Design review of the part built by this model. Coordinates are the model's own, in mm. Face numbers are marked on the shaded views. A direction names the side the tool comes from. Give positions to 0.01 mm unless a question says otherwise; leave off trailing zeros. Write each loop counter-clockwise with the first axis right and the second up, starting at its lowest first coordinate (ties: lowest second). Pieces come first, ordered by that corner, then holes. Notation, with made-up numbers: (69, 37) -> (113, 37) arc R32 cw to (113, 75) -> close; hole circle Ø5 at (60.25, 86). An arc over 180 degrees is marked (long way). Use CSV: the item, a comma, the result in double quotes.
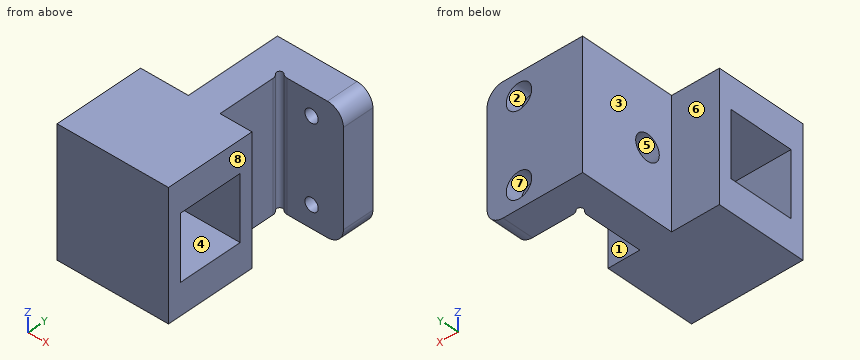
```python
from build123d import *

# Parameters (mm, degrees)
DODANIE_WYCI_GNI_CIE1_DEPTH = 40
SZKIC7_R                    = 4
WYTNIJ_WYCI_GNI_CIE2_DEPTH  = 5
SZKIC8_R                    = 2.1
WYTNIJ_WYCI_GNI_CIE3_DEPTH  = 5
SZKIC9_R                    = 4
WYTNIJ_WYCI_GNI_CIE4_DEPTH  = 5
SZKIC10_R                   = 2.1
WYTNIJ_WYCI_GNI_CIE5_DEPTH  = 5
ZAOKR_GLENIE1_R             = 5
BOSS_EXTRUDE1_DEPTH         = 15
BOSS_EXTRUDE1_DEPTH_BACK    = 20.0001
SKETCH1_W                   = 40
SKETCH1_H                   = 28.3
SKETCH1_W_2                 = 20.3
SKETCH1_H_2                 = 20.3


with BuildPart() as part:
    # Szkic1 → Dodanie-wyciągnięcie1 (new body)
    with BuildSketch(Plane.XY):
        with BuildLine():
            Line((0, 0), (0, 19.763932023))
            ThreePointArc((0, 19.763932023), (-0.174258142, 20.580428603), (-0.666666667, 21.254644008))
            ThreePointArc((-0.666666667, 21.254644008), (-0.707106781, 22.707106781), (0.745355992, 22.666666667))
            ThreePointArc((0.745355992, 22.666666667), (1.419571397, 22.174258142), (2.236067977, 22))
            Line((2.236067977, 22), (20, 22))
            Line((20, 22), (20, 32))
            Line((20, 32), (-10, 32))
            Line((-10, 32), (-10, 0))
            Line((-10, 0), (0, 0))
        make_face()
    extrude(amount=DODANIE_WYCI_GNI_CIE1_DEPTH)

    # Szkic7 → Wytnij-wyciągnięcie2 (cut)
    with BuildSketch(Plane.ZY.offset(10)):
        with Locations(Location((20, 10, 0), (0, 0, 270))):
            Circle(SZKIC7_R)
    extrude(amount=-WYTNIJ_WYCI_GNI_CIE2_DEPTH, mode=Mode.SUBTRACT)

    # Szkic8 → Wytnij-wyciągnięcie3 (cut)
    with BuildSketch(Plane.ZY.offset(5)):
        with Locations(Location((20, 10, 0), (0, 0, 270))):
            Circle(SZKIC8_R)
    extrude(amount=-WYTNIJ_WYCI_GNI_CIE3_DEPTH, mode=Mode.SUBTRACT)

    # Szkic9 → Wytnij-wyciągnięcie4 (cut)
    with BuildSketch(Plane(origin=(0, 32, 0), x_dir=(1, 0, 0), z_dir=(0, 1, 0))):
        with Locations(Location((10, -33, 0), (0, 0, 180))):
            Circle(SZKIC9_R)
        with Locations(Location((10, -7, 0), (0, 0, 180))):
            Circle(SZKIC9_R)
    extrude(amount=-WYTNIJ_WYCI_GNI_CIE4_DEPTH, mode=Mode.SUBTRACT)

    # Szkic10 → Wytnij-wyciągnięcie5 (cut)
    with BuildSketch(Plane(origin=(0, 27, 0), x_dir=(1, 0, 0), z_dir=(0, 1, 0))):
        with Locations(Location((10, -33, 0), (0, 0, 180))):
            Circle(SZKIC10_R)
        with Locations(Location((10, -7, 0), (0, 0, 180))):
            Circle(SZKIC10_R)
    extrude(amount=-WYTNIJ_WYCI_GNI_CIE5_DEPTH, mode=Mode.SUBTRACT)

    # Zaokrąglenie1
    zaokr_glenie1_edges = [part.edges().sort_by_distance(p)[0] for p in [
        (20, 27, 0),
        (20, 27, 40),
    ]]
    fillet(zaokr_glenie1_edges, radius=ZAOKR_GLENIE1_R)

    # Sketch1 → Boss-Extrude1 (add, two sides: drawn at the far end of the back side and taken through both)
    with BuildSketch(Plane.ZY.offset(10).offset(-BOSS_EXTRUDE1_DEPTH_BACK)):
        with Locations((20, -12.35)):
            Rectangle(SKETCH1_W, SKETCH1_H)
        with Locations((20, -12.35)):
            Rectangle(SKETCH1_W_2, SKETCH1_H_2, mode=Mode.SUBTRACT)
    extrude(amount=BOSS_EXTRUDE1_DEPTH + BOSS_EXTRUDE1_DEPTH_BACK)


solid = part.part
```
(1) Tool access review of the marked faces 1, 2, 3, 4 and 5: name each direction out of +Z, -Z, +X, -X, +Y, -Y from which nothing blocks a thin tool from reaching the whole face with its end or side.
Established:
face 1,"+Z, -Z, +X"
face 2,"+Y"
face 3,"+Z, -Z, -X, +Y"
face 4,"+X, -X"
face 5,"-X"
(2) For line 1 along Z through (x, y) = (10, 29.9); line 2 along Z through (x, y) = (7, -11.5); line 3 along Z through (x, y) = (-7.45, 10), list the stretches that pass through material, from the lowest coordinate up. Write a range as [from, to].
Established:
line 1,"z = [0, 3], [11, 29], [37, 40]"
line 2,"z = [0, 9.85], [30.15, 40]"
line 3,"z = [0, 16], [24, 40]"
(3) Take a section at D-D (x = -12). Write out the cut boundary in (y, z).
Established:
outline,"(-26.5, 0) -> (1.8, 0) -> (1.8, 40) -> (-26.5, 40) -> close; hole (-22.5, 9.85) -> (-2.2, 9.85) -> (-2.2, 30.15) -> (-22.5, 30.15) -> close"
(4) Clearance check with flat-ended pins moving along their axes: pin 1 (8.5 mm diameter, centred on y = -13.5, z = 29.5, fed in from +X); pin 2 (4 mm diameter, centred on y = 11.5, z = 19, fed in from -X); pin 3 (2.5 mm diameter, centred on x = 9.5, z = 6.5, fed in from +Y); pin 4 (2 mm diameter, centred on y = -7, z = 11, fed in from +X). State where each tip first meets the part, or that it passes through.
Established:
pin 1,"stops at x = 10"
pin 2,"stops at x = -5"
pin 3,"stops at y = 1.8"
pin 4,"passes through"
(5) Mouldability with a two-part tool opening along X and no side actions: class the marked faces 6, 7 and 8 as +X half, -X half, draft (parallel to the pull), parting line (faces both ways), or undercut.
Established:
face 6,"draft"
face 7,"undercut"
face 8,"+X half"
(6) Take a section at A-A (x = 3). Write out the cut boundary in (y, z), then the cut area to 3 significant figures.
Established:
outline,"(-26.5, 0) -> (1.8, 0) -> (1.8, 40) -> (-26.5, 40) -> close; (22, 0) -> (32, 0) -> (32, 40) -> (22, 40) -> close; hole (-22.5, 9.85) -> (-2.2, 9.85) -> (-2.2, 30.15) -> (-22.5, 30.15) -> close"
area,"1,120 mm2"
(7) Take a section at B-B (z = 26). Write out the cut boundary in (x, y), then the cut area to 3 significant figures.
Established:
outline,"(-25, -26.5) -> (10, -26.5) -> (10, -22.5) -> (-25, -22.5) -> close; (-25, -2.2) -> (10, -2.2) -> (10, 1.8) -> (0, 1.8) -> (0, 19.76) arc R2 ccw to (-0.67, 21.25) arc R1 cw (long way) to (0.75, 22.67) arc R2 ccw to (2.24, 22) -> (20, 22) -> (20, 32) -> (-10, 32) -> (-10, 1.8) -> (-25, 1.8) -> close"
area,"779 mm2"
(8) Take a section at C-C (y = -4.5). Write out the cut boundary in (x, z).
Established:
outline,"(-25, 0) -> (10, 0) -> (10, 9.85) -> (-25, 9.85) -> close; (-25, 30.15) -> (10, 30.15) -> (10, 40) -> (-25, 40) -> close"
